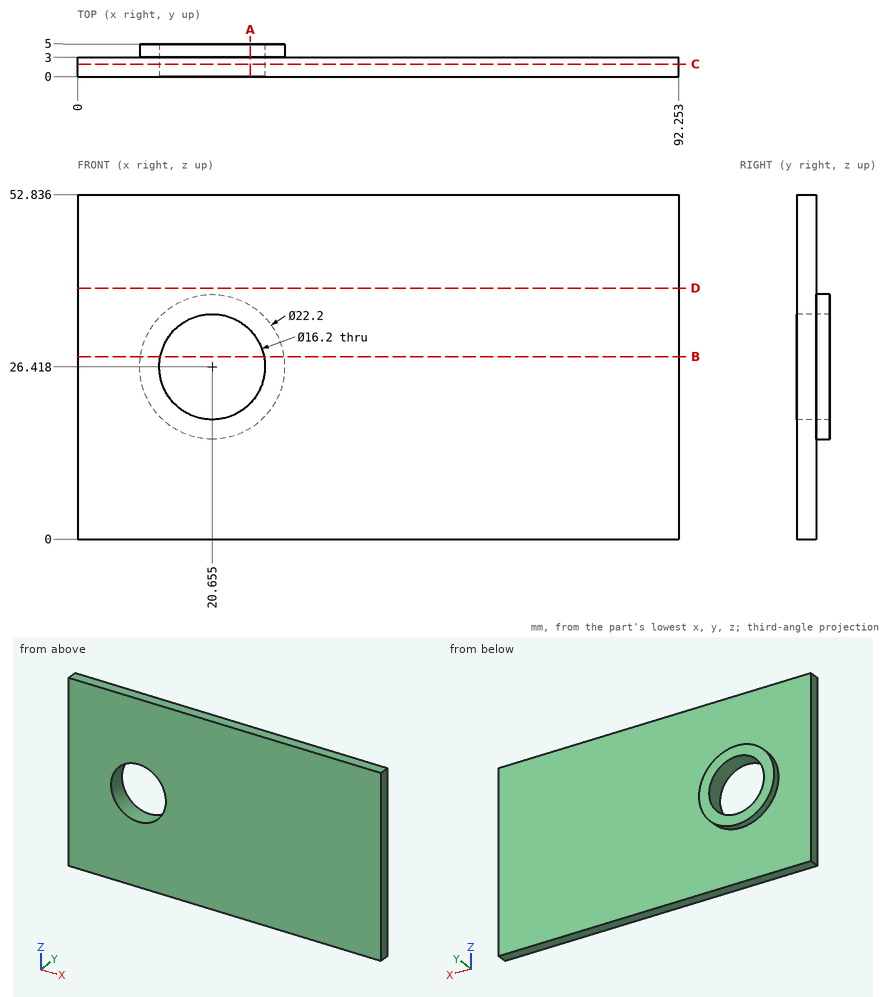
Here's the drawing with two shaded views (mm, measured from the low corner). I have some questions. Give positions to 0.01 mm unless a question says otherwise; leave off trailing zeros. Loops run counter-clockwise (first coordinate to the right, second up) from the corner with the lowest first, then second, coordinate; pieces in that order, holes last. Notation, with made-up numbers: M 24.25,12.25 L 43.25,12.25 A23 cw 43.25,44.25 Z; hole C 54.5,53 d5. An arc over 180 degrees is marked long. Use one line per item in the form item = value. Start each with the question number.
(1) I'm going to push flat-ended pins straight in: P1, Ø4, axis at x = 75, z = 34, coming from the -Y side; P2, Ø5, axis at x = 80, z = 13.5, coming from the +Y side. Where does each tip first touch, or does it pass through?
(2) Please list where these lines run through material, in increasing order: line 1 (X direction, y = 2.95, z = 26.5) (1 decimal); line 2 (Y direction, x = 32.5, z = 42); line 3 (X direction, y = 1.1, z = 25.5).
(3) I want a section at A-A, the plane x = 26.5. Write out the boundary of the cut face in (y, z) (1 decimal).
(4) I want a section at C-C, the plane y = 1.9. Write out the boundary of the cut face in (x, z) (1 decimal), and give its area (3 significant figures).
(5) I want a section at D-D, the plane z = 38.5. Write out the boundary of the cut face in (x, y).
(6) I want a section at B-B, the plane z = 28. Write out the boundary of the cut face in (x, y).
Worked out:
q1.P1 = 0
q1.P2 = 3
q2.line_1 = 0 to 12.6, 28.8 to 92.3
q2.line_2 = 0 to 3
q2.line_3 = 0 to 12.61, 28.7 to 92.25
q3.outline = M 0,0 L 3,0 L 3,17 L 5,17 L 5,20.8 L 0,20.8 Z; M 0,32 L 5,32 L 5,35.9 L 3,35.9 L 3,52.8 L 0,52.8 Z
q4.outline = M 0,0 L 92.3,0 L 92.3,52.8 L 0,52.8 Z; hole C 20.7,26.4 d16.2
q4.area = 4,670 mm²
q5.outline = M 0,0 L 92.25,0 L 92.25,3 L 0,3 Z
q6.outline = M 0,0 L 12.71,0 L 12.71,5 L 9.67,5 L 9.67,3 L 0,3 Z; M 28.6,0 L 92.25,0 L 92.25,3 L 31.64,3 L 31.64,5 L 28.6,5 Z
